```python
from build123d import *
from OCP.BRepFilletAPI import BRepFilletAPI_MakeChamfer

# Parameters (mm, degrees)
SKETCH4_R          = 2.6
SKETCH4_R_2        = 3.1
CUT_EXTRUDE1_DEPTH = 5.2
SKETCH5_W          = 9.9
SKETCH5_H          = 6
SKETCH5_W_2        = 9.5
CUT_EXTRUDE2_DEPTH = 82
FILLET3_R          = 2
CHAMFER1_SIZE      = 1
CHAMFER1_SIZE2     = 1.191753593
CUT_EXTRUDE3_DEPTH = 90.2
FILLET4_R          = 0.2
FILLET5_R          = 0.5


with BuildPart() as part:
    # Sketch1 → Loft1 section 0
    with BuildSketch(Plane.XY):
        with BuildLine():
            add(Edge.make_bspline(
                [(115, 0), (114.999913382, 0.00327866), (114.222934603, -0.004567066), (113.418136575, 0.000318408), (111.44543546, 0.018706002), (108.999380922, 0.080565277), (105.780115155, 0.203144323), (101.978037922, 0.467320429), (97.63148646, 0.880990765), (92.843812566, 1.427373326), (87.693014802, 2.062174327), (82.26127365, 2.794917392), (76.628898252, 3.582200475), (70.875421432, 4.408274793), (65.069516957, 5.204495648), (59.272555938, 5.964988559), (53.535411353, 6.612069385), (47.902032041, 7.147901639), (42.420677472, 7.538059951), (37.125743857, 7.784294524), (32.060080889, 7.863888962), (27.260899934, 7.799703202), (22.764274035, 7.585443948), (18.606628598, 7.224009749), (14.819582747, 6.717397261), (11.43119341, 6.102885155), (8.463318021, 5.359495242), (5.929953708, 4.523167874), (3.840235227, 3.611431652), (2.203139301, 2.680524392), (0.997143498, 1.719388226), (0.306055902, 0.84473605), (-0.153897847, -0.016785493), (0.441131195, -0.783771302), (1.630250645, -0.976182526), (3.345026164, -1.247099953), (5.741349663, -1.385446358), (8.741002332, -1.531007587), (12.32356917, -1.613427576), (16.426146399, -1.711956772), (20.996614723, -1.764001286), (25.979915364, -1.804105207), (31.316658928, -1.826220598), (36.950031377, -1.811871436), (42.810070502, -1.783755804), (48.833365319, -1.730024981), (54.950109545, -1.67348399), (61.093513049, -1.595166549), (67.193299365, -1.488121719), (73.176935484, -1.397778739), (78.980025922, -1.271232402), (84.533413271, -1.152999753), (89.776869938, -1.037364871), (94.647010434, -0.905039683), (99.089599698, -0.778312882), (103.055602703, -0.646322839), (106.488295637, -0.529569147), (109.391284428, -0.370730171), (111.629000068, -0.244208643), (113.467096811, -0.099576309), (114.237158295, -0.036931621), (115.000086752, -0.003283716), (115, 0)],
                knots=[0, 0, 0, 0, 0.001545172, 0.006223608, 0.014035782, 0.024855049, 0.038644124, 0.055163693, 0.074045466, 0.094820373, 0.117222732, 0.140866367, 0.165395395, 0.190452399, 0.215710088, 0.240854358, 0.265734023, 0.290048364, 0.313714428, 0.336486101, 0.358292895, 0.378940292, 0.398278007, 0.416246563, 0.432660408, 0.447459903, 0.460566131, 0.472021733, 0.481783695, 0.489844359, 0.496307136, 0.50126117, 0.504695153, 0.507385543, 0.512190444, 0.519692984, 0.529980259, 0.542956454, 0.558414131, 0.576101982, 0.595804604, 0.61726601, 0.64027206, 0.66452271, 0.689803764, 0.7157292, 0.742084221, 0.768568973, 0.794840399, 0.820639753, 0.845625339, 0.869581038, 0.892163588, 0.913159587, 0.932310678, 0.94940252, 0.964220925, 0.976641917, 0.986532119, 0.993892864, 0.998452446, 1, 1, 1, 1], degree=3))
        make_face()
    # Sketch2 → Loft1 section 1
    with BuildSketch(Plane.XY.offset(-120)):
        with BuildLine():
            add(Edge.make_bspline(
                [(110, 0), (110.000464145, 0.002638021), (109.253557002, -0.006421882), (108.485306247, 0.00202473), (106.599515685, 0.014018922), (104.259903283, 0.071192731), (101.178986874, 0.200889618), (97.542661477, 0.451950761), (93.384633146, 0.843539364), (88.805204424, 1.362015696), (83.880374164, 1.978555721), (78.68657223, 2.677523385), (73.299477431, 3.430735281), (67.795235431, 4.215247142), (62.241233075, 4.984660857), (56.695525551, 5.697469803), (51.207787306, 6.322755672), (45.821489693, 6.833626486), (40.577824462, 7.211562863), (35.514283248, 7.444282984), (30.668486135, 7.527509184), (26.076763803, 7.463490784), (21.77566696, 7.255221358), (17.798933432, 6.909184212), (14.177047879, 6.430194992), (10.935139134, 5.831964767), (8.094704102, 5.122344568), (5.670248347, 4.327180111), (3.669790047, 3.460558372), (2.10909167, 2.56151381), (0.952680778, 1.647952784), (0.292493833, 0.810328248), (-0.144477468, -0.013443729), (0.421457768, -0.751792674), (1.561430619, -0.927732015), (3.196411713, -1.199647616), (5.489901797, -1.325203312), (8.359384575, -1.457341268), (11.786506209, -1.55318322), (15.712038629, -1.632817261), (20.085890157, -1.693490267), (24.85332264, -1.730533844), (29.958495668, -1.745317698), (35.344133299, -1.736641885), (40.949025669, -1.70754651), (46.710109342, -1.660092686), (52.562107594, -1.595708584), (58.438334584, -1.519615465), (64.272360823, -1.429130605), (69.997133878, -1.329443239), (75.548112692, -1.222377083), (80.861507128, -1.10840335), (85.876724326, -0.990587124), (90.536246874, -0.869398239), (94.784781842, -0.746694986), (98.577741113, -0.621781265), (101.858350076, -0.496229968), (104.635869759, -0.366297292), (106.773720091, -0.224338993), (108.53252638, -0.099668194), (109.269457647, -0.031974616), (109.999539654, -0.002616432), (110, 0)],
                knots=[0, 0, 0, 0, 0.001564721, 0.006239121, 0.014018617, 0.024861007, 0.038659987, 0.055174427, 0.074046407, 0.094837256, 0.117226118, 0.14085626, 0.165386109, 0.19045125, 0.215702393, 0.240866612, 0.265718976, 0.290051983, 0.313696202, 0.33648442, 0.358279861, 0.378929437, 0.398292398, 0.416235766, 0.432650472, 0.447455618, 0.460592079, 0.472030369, 0.48177877, 0.489853088, 0.496315276, 0.501246195, 0.504684904, 0.507403743, 0.512183233, 0.519672773, 0.529968131, 0.54294809, 0.558399818, 0.576099165, 0.595810572, 0.617282889, 0.64027984, 0.664535393, 0.689783385, 0.715732831, 0.742092653, 0.768566703, 0.794844175, 0.820638712, 0.845644257, 0.86958445, 0.892182833, 0.913177877, 0.932327829, 0.949410904, 0.964230176, 0.976629486, 0.986536787, 0.993881551, 0.998448084, 1, 1, 1, 1], degree=3))
        make_face()
    loft()

    # Sketch4 → Cut-Extrude1 (cut)
    with BuildSketch(Plane.XY):
        with Locations((10.5, 2)):
            Circle(SKETCH4_R)
        with Locations((57, 2.1)):
            Circle(SKETCH4_R_2)
    extrude(amount=-CUT_EXTRUDE1_DEPTH, mode=Mode.SUBTRACT)

    # Sketch5 → Cut-Extrude2 (cut)
    with BuildSketch(Plane.XY):
        with Locations((21, 2.8)):
            Rectangle(SKETCH5_W, SKETCH5_H)
        with Locations((46, 3)):
            Rectangle(SKETCH5_W_2, SKETCH5_H)
    extrude(amount=-CUT_EXTRUDE2_DEPTH, mode=Mode.SUBTRACT)

    # Fillet3
    fillet3_edges = [part.edges().sort_by_distance(p)[0] for p in [
        (25.95, 5.8, -41),
        (16.05, 5.8, -41),
        (50.75, 6, -41),
        (41.25, 6, -41),
    ]]
    fillet(fillet3_edges, radius=FILLET3_R)

    # Chamfer1: one chamfer whose edges measure the first distance from different faces: ONE call of the kernel's chamfer builder (chamfer() names one face for all edges)
    chamfer1_edges_1 = [part.edges().sort_by_distance(p)[0] for p in [
        (25.95, -0.2, -41),
    ]]
    chamfer1_side_1 = [part.faces().sort_by_distance(p)[0] for p in [
        (21, -0.2, -41),
    ]]
    chamfer1_edges_2 = [part.edges().sort_by_distance(p)[0] for p in [
        (16.05, -0.2, -41),
    ]]
    chamfer1_side_2 = [part.faces().sort_by_distance(p)[0] for p in [
        (16.05, 1.8, -41),
    ]]
    chamfer1_edges_3 = [part.edges().sort_by_distance(p)[0] for p in [
        (50.75, 0, -41),
    ]]
    chamfer1_side_3 = [part.faces().sort_by_distance(p)[0] for p in [
        (46, 0, -41),
    ]]
    chamfer1_edges_4 = [part.edges().sort_by_distance(p)[0] for p in [
        (41.25, 0, -41),
    ]]
    chamfer1_side_4 = [part.faces().sort_by_distance(p)[0] for p in [
        (41.25, 2, -41),
    ]]
    chamfer1 = BRepFilletAPI_MakeChamfer(part.part.solid().wrapped)
    for e in chamfer1_edges_1:
        chamfer1.Add(CHAMFER1_SIZE, CHAMFER1_SIZE2, e.wrapped, chamfer1_side_1[0].wrapped)  # the first distance lies on this face
    for e in chamfer1_edges_2:
        chamfer1.Add(CHAMFER1_SIZE, CHAMFER1_SIZE2, e.wrapped, chamfer1_side_2[0].wrapped)  # the first distance lies on this face
    for e in chamfer1_edges_3:
        chamfer1.Add(CHAMFER1_SIZE, CHAMFER1_SIZE2, e.wrapped, chamfer1_side_3[0].wrapped)  # the first distance lies on this face
    for e in chamfer1_edges_4:
        chamfer1.Add(CHAMFER1_SIZE, CHAMFER1_SIZE2, e.wrapped, chamfer1_side_4[0].wrapped)  # the first distance lies on this face
    add(Compound.cast(chamfer1.Shape()), mode=Mode.REPLACE)

    # Sketch6 → Cut-Extrude3 (cut)
    with BuildSketch(Plane.XY):
        Polygon((62.411905862, 3.940649629), (62.411905862, 0), (91.123097262, 0.343480777), align=None)
    extrude(amount=-CUT_EXTRUDE3_DEPTH, mode=Mode.SUBTRACT)

    # Fillet4
    fillet4_edges = [part.edges().sort_by_distance(p)[0] for p in [
        (91.123097262, 0.343480777, -45.1),
    ]]
    fillet(fillet4_edges, radius=FILLET4_R)

    # Fillet5
    fillet5_edges = [part.edges().sort_by_distance(p)[0] for p in [
        (62.411905862, 0, -45.1),
        (62.411905862, 3.940649629, -45.1),
    ]]
    fillet(fillet5_edges, radius=FILLET5_R)


solid = part.part
```
The listing builds one solid part. Answer for the finished solid, in the listing's coordinates (mm). A direction names the side the tool comes from. Round coordinates to 2 decimals unless told otherwise and drop trailing zeros. Return JSON: item names as keys, results as strings. Group by question number.
1. Which of the six approach directions +Z, -Z, +X, -X, +Y, -Y give full straight-line access (tool end or side, diameter ignored) to faces 1 (the flat face through (43, 2, -120)), 2 (the flat face through (46, 3, -82))?
2. The mould has two halves that part along Y. Classify faces 3 (the flat face through (45, -1, 0)), 4 (the flat face through (16.05, 2, -40)): pulls with the +Y half, pulls with the -Y half, needs draft (parallel to the pull), parting line crosses it, or undercut.
3. Each of these flat-tipped pins is pushed along its axis until it touches: P1, Ø5, axis at x = 102.5, y = 4, coming from the +Z side; P2, Ø3.5, axis at x = 57, y = 2.1, coming from the +Z side; P3, Ø1.4, axis at y = 3, z = -48.5, coming from the -X side; P4, Ø8, axis at x = 44.5, z = -65.5, coming from the +Y side. Where does it stop, or does it pass through?
4. Consider probe 1 along Y at (x, z) = (23, -64.5); probe 2 along Y at (x, z) = (10.5, -2.2); probe 3 along Z at (x, y) = (50, 2). Determine where each line is inside the solid, lowest interval first.
Resolved:
{
 "1": {"face 1": "-Z, +X, -X, +Y, -Y", "face 2": "+Z"},
 "2": {"face 3": "needs draft", "face 4": "undercut"},
 "3": {"P1": "passes through", "P2": "stops at z = -5.2", "P3": "stops at x = 1.77", "P4": "stops at y = 7.39"},
 "4": {"probe 1": "y = -1.74 to -0.2, 5.8 to 7.43", "probe 2": "y = -1.57 to -0.6, 4.6 to 5.85", "probe 3": "z = -120 to -82"}
}
